Could you check a few things on this model? Use its own coordinates, in mm. Round coordinates to 2 decimals unless told otherwise and drop trailing zeros. Loops run counter-clockwise (first coordinate to the right, second up) from the corner with the lowest first, then second, coordinate; pieces in that order, holes last. Notation, with made-up numbers: (4.25, 30) - (26.25, 30) arc R22 ccw to (26.25, 50) - close; hole circle Ø8 at (16.25, 74). An arc over 180 degrees is marked (long way). Answer as CSV lines item,"result". Start each with the question number.
1) Suppose I cut it at A-A, the plane x = 176.3. Write out the boundary of the cut face in (y, z), then the cut area to 3 significant figures.
2) Suppose I cut it at D-D, the plane y = 53. Write out the boundary of the cut face in (x, z).
3) Suppose I cut it at B-B, the plane y = 18. Write out the boundary of the cut face in (x, z) (3 decimals), then the cut area to 3 significant figures.
4) Please list where these lines run through material, in increasing order: line 1 along Y through (x, z) = (161.3, 0.4) (3 decimals); line 2 along X through (y, z) = (28.5, 1); line 3 along Y through (x, z) = (53, 0.3).
5) I'm going to push a flat-ended pin straight in: pin 1 Ø0.5 at (x, z) = (62, 0.5) entering from -Y. Where does the tip first touch, or does it pass through?
6) Suppose I cut it at C-C, the plane z = 1.05. Write out the boundary of the cut face in (x, y) (3 decimals), then the cut area to 3 significant figures.
```python
from build123d import *

# Parameters (mm, degrees)
SKETCH_W      = 191.3
SKETCH_H      = 68
PAD_DEPTH     = 1.65
SKETCH001_R   = 4.05
SKETCH001_R_2 = 3
SKETCH001_R_3 = 3.175
SKETCH001_W   = 20
SKETCH001_H   = 5
POCKET_DEPTH  = 5


with BuildPart() as part:
    # Sketch → Pad (new body)
    with BuildSketch(Plane.XY):
        with Locations((95.65, 34)):
            Rectangle(SKETCH_W, SKETCH_H)
    extrude(amount=PAD_DEPTH)

    # Sketch001 (on Face6 of Pad) → Pocket (cut)
    with BuildSketch(Plane.XY.offset(1.65)):
        with Locations((176.3, 53)):
            Circle(SKETCH001_R)
        with Locations((121.3, 18)):
            Circle(SKETCH001_R_2)
        with Locations((146.3, 18)):
            Circle(SKETCH001_R_3)
        with Locations((161.3, 18)):
            Circle(SKETCH001_R_3)
        with Locations((60, 29.5)):
            Rectangle(SKETCH001_W, SKETCH001_H)
    extrude(amount=-POCKET_DEPTH, mode=Mode.SUBTRACT)


solid = part.part
```
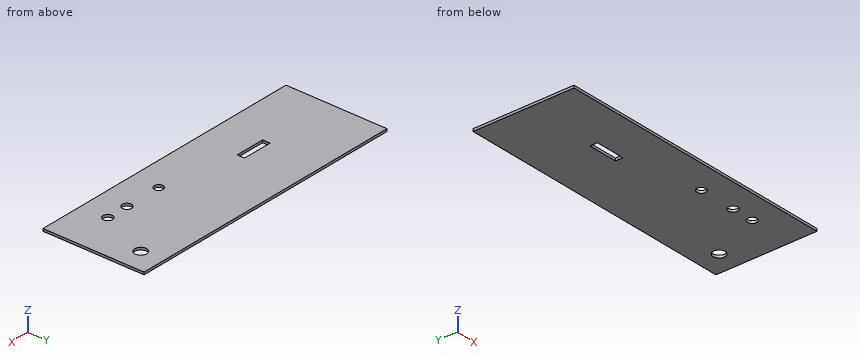
Filled sheet:
1,outline,"(0, 0) - (48.95, 0) - (48.95, 1.65) - (0, 1.65) - close; (57.05, 0) - (68, 0) - (68, 1.65) - (57.05, 1.65) - close"
1,area,"98.8 mm²"
2,outline,"(0, 0) - (172.25, 0) - (172.25, 1.65) - (0, 1.65) - close; (180.35, 0) - (191.3, 0) - (191.3, 1.65) - (180.35, 1.65) - close"
3,outline,"(0, 0) - (118.3, 0) - (118.3, 1.65) - (0, 1.65) - close; (124.3, 0) - (143.125, 0) - (143.125, 1.65) - (124.3, 1.65) - close; (149.475, 0) - (158.125, 0) - (158.125, 1.65) - (149.475, 1.65) - close; (164.475, 0) - (191.3, 0) - (191.3, 1.65) - (164.475, 1.65) - close"
3,area,"285 mm²"
4,line 1,"0 to 14.825, 21.175 to 68"
4,line 2,"0 to 50, 70 to 191.3"
4,line 3,"0 to 27, 32 to 68"
5,pin 1,"y = 0"
6,outline,"(0, 0) - (191.3, 0) - (191.3, 68) - (0, 68) - close; hole (50, 27) - (70, 27) - (70, 32) - (50, 32) - close; hole circle Ø6 at (121.3, 18); hole circle Ø6.35 at (146.3, 18); hole circle Ø6.35 at (161.3, 18); hole circle Ø8.1 at (176.3, 53)"
6,area,"12,800 mm²"
